Verification items for the finished model (mm, model axes). A direction names the side the tool comes from. Round coordinates to 2 decimals unless told otherwise and drop trailing zeros. Order: outer loops, then holes, each group sorted by start corner. A loop starts at its lowest first (then second) coordinate and runs counter-clockwise, first axis right, second up. Notation, with made-up numbers: (89, -14) -> (138, -14) arc R20 cw to (138, 4) -> close; hole circle Ø5 at (72, 81.25). An arc over 180 degrees is marked (long way). Return JSON: item names as keys, results as strings. Group by question number.
Item 1: Access from +Z, -Z, +X, -X, +Y, -Y to the whole of each face (thin tool, end or side, straight path). Record for faces 4 (the cylindrical face through (31.843, 2.465, -8.381)), 5 (the flat face through (-37, 2, 6)), 6 (the flat face through (-26, 2, -0.875)).
Item 2: Sectioned sample at A-A on x = -42. Record the cut outline in (y, z) (3 decimals).
Item 3: Sectioned sample at C-C on x = -31. Record the cut outline in (y, z) (3 decimals), plus the area to 3 significant figures.
Item 4: Draft check along X on faces 1 (the cylindrical face through (4.696, 2.465, -0.002)), 2 (the flat face through (-41, 3, 8.125)), 3 (the flat face through (-45, 2, -2)). Enter one of: pulls with the +X half, pulls with the -X half, needs draft (parallel to the pull), parting line crosses it, or undercut.
Item 5: Sectioned sample at B-B on y = 1.95. Give the number of separate pieces and of enclosed holes in the cut face, plus the area to 3 significant figures.
Item 6: Depth check by flat-ended pin: pin 1 Ø1.3 at (x, y) = (34.5, 3) entering from +Z (3 decimals). Enter the tip coordinate at first touch or a pass-through.
Item 7: Sectioned sample at D-D on z = -6.5. Record the cut outline in (x, y), plus the area to 3 significant figures.
Item 8: Scan lines: probe 1 along Z at (x, y) = (-27.5, 2.2) (3 decimals); probe 2 along X at (y, z) = (3.95, 7.25); probe 3 along X at (y, z) = (3.5, 4.5). Record each from-to range of solid material in increasing order. Write a range as from..to.
```python
from build123d import *

# Parameters (mm, degrees)
BOSS_EXTRUDE1_DEPTH = 5
SKETCH2_W           = 8
SKETCH2_H           = 5
BOSS_EXTRUDE2_DEPTH = 9
FILLET1_R           = 4
SKETCH3_R           = 1.5
CUT_EXTRUDE1_DEPTH  = 10


with BuildPart() as part:
    # Sketch1 → Boss-Extrude1 (new body)
    with BuildSketch(Plane.XZ):
        with BuildLine():
            Line((-45, -0.875), (-45, -11.375))
            Line((-45, -11.375), (24.5, -11.375))
            ThreePointArc((24.5, -11.375), (31.924621202, -8.299621202), (35, -0.875))
            Line((35, -0.875), (33.775, -0.875))
            ThreePointArc((33.775, -0.875), (30.670128687, -0.026396946), (27.825, -1.531586558))
            ThreePointArc((27.825, -1.531586558), (24.5, 0), (21.175, -1.531586558))
            ThreePointArc((21.175, -1.531586558), (17.85, 0), (14.525, -1.531586558))
            ThreePointArc((14.525, -1.531586558), (11.2, 0), (7.875, -1.531586558))
            ThreePointArc((7.875, -1.531586558), (4.55, 0), (1.225, -1.531586558))
            ThreePointArc((1.225, -1.531586558), (-2.1, 0), (-5.425, -1.531586558))
            ThreePointArc((-5.425, -1.531586558), (-8.861439615, -0.00141952), (-12.215492713, -1.704609531))
            ThreePointArc((-12.215492713, -1.704609531), (-15.090502578, -0.040031141), (-18.305985425, -0.875))
            Line((-18.305985425, -0.875), (-45, -0.875))
        make_face()
    extrude(amount=-BOSS_EXTRUDE1_DEPTH)

    # Sketch2 → Boss-Extrude2 (add)
    with BuildSketch(Plane.XY.offset(-0.875)):
        with Locations((-41, 2.5)):
            Rectangle(SKETCH2_W, SKETCH2_H)
    extrude(amount=BOSS_EXTRUDE2_DEPTH)

    # Chamfer1
    # the kernel refuses this chamfer: 0.5, 0.339586842 mm, written as the material it adds along each edge
    with BuildSketch(Plane(origin=(-5.425, 0, -1.531586558), x_dir=(0.6961293101624768, 0, 0.7179164182080768), z_dir=(0, 1, 0))) as chamfer1_piece_1:
        with BuildLine():
            Line((0.546593526, 0), (0.018611268, -0.34666682))
            ThreePointArc((0.018611268, -0.34666682), (0.013013217, -0.178188087), (0, 0))
            ThreePointArc((0, 0), (0.281682829, -0.008536435), (0.546593526, 0))
        make_face()
    extrude(amount=5)
    with BuildSketch(Plane(origin=(1.225, 0, -1.531586558), x_dir=(-0.6795651691098796, 0, 0.7336151449722536), z_dir=(0, 1, 0)), Plane(origin=(7.875, 0, -1.531586558), x_dir=(-0.67956516910988, 0, 0.7336151449722534), z_dir=(0, 1, 0)), Plane(origin=(14.525, 0, -1.531586558), x_dir=(-0.679565169109884, 0, 0.7336151449722498), z_dir=(0, 1, 0)), Plane(origin=(21.175, 0, -1.531586558), x_dir=(-0.6795651691098812, 0, 0.7336151449722523), z_dir=(0, 1, 0)), Plane(origin=(27.825, 0, -1.531586558), x_dir=(-0.6795651691098773, 0, 0.7336151449722558), z_dir=(0, 1, 0))) as chamfer1_piece_2:
        with BuildLine():
            Line((0.347166046, 0), (0.029302401, 0.545807522))
            ThreePointArc((0.029302401, 0.545807522), (0.023624929, 0.280820137), (0, 0))
            ThreePointArc((0, 0), (0.178629479, 0.003441996), (0.347166046, 0))
        make_face()
    extrude(amount=5)

    # Fillet1
    fillet1_edges = [part.edges().sort_by_distance(p)[0] for p in [
        (-37, 2.5, -0.875),
    ]]
    fillet(fillet1_edges, radius=FILLET1_R)

    # Sketch3 → Cut-Extrude1 (cut)
    with BuildSketch(Plane(origin=(0, 5, 0), x_dir=(1, 0, 0), z_dir=(0, 1, 0))):
        with Locations(Location((-42, -5.125, 0), (0, 0, 270))):
            Circle(SKETCH3_R)
        with Locations(Location((-42, 8.875, 0), (0, 0, 270))):
            Circle(SKETCH3_R)
    extrude(amount=-CUT_EXTRUDE1_DEPTH, mode=Mode.SUBTRACT)


solid = part.part
```
Recorded:
{
 "1": {"face 4": "-Z, +X, +Y, -Y", "face 5": "+Z, +X, +Y, -Y", "face 6": "+Z, +Y, -Y"},
 "2": {"outline": "(0, -11.375) -> (5, -11.375) -> (5, -10.375) -> (0, -10.375) -> close; (0, -7.375) -> (5, -7.375) -> (5, 3.625) -> (0, 3.625) -> close; (0, 6.625) -> (5, 6.625) -> (5, 8.125) -> (0, 8.125) -> close"},
 "3": {"outline": "(0, -11.375) -> (5, -11.375) -> (5, -0.875) -> (0, -0.875) -> close", "area": "52.5 mm²"},
 "4": {"face 1": "undercut", "face 2": "needs draft", "face 3": "pulls with the -X half"},
 "5": {"separate pieces": "1", "enclosed holes": "2", "area": "900 mm²"},
 "6": {"pin 1": "z = -0.875"},
 "7": {"outline": "(-45, 0) -> (33.37, 0) -> (33.37, 5) -> (-45, 5) -> close", "area": "392 mm²"},
 "8": {"probe 1": "-11.375..-0.875", "probe 2": "-45..-37", "probe 3": "-45..-43.36, -40.64..-37"}
}
